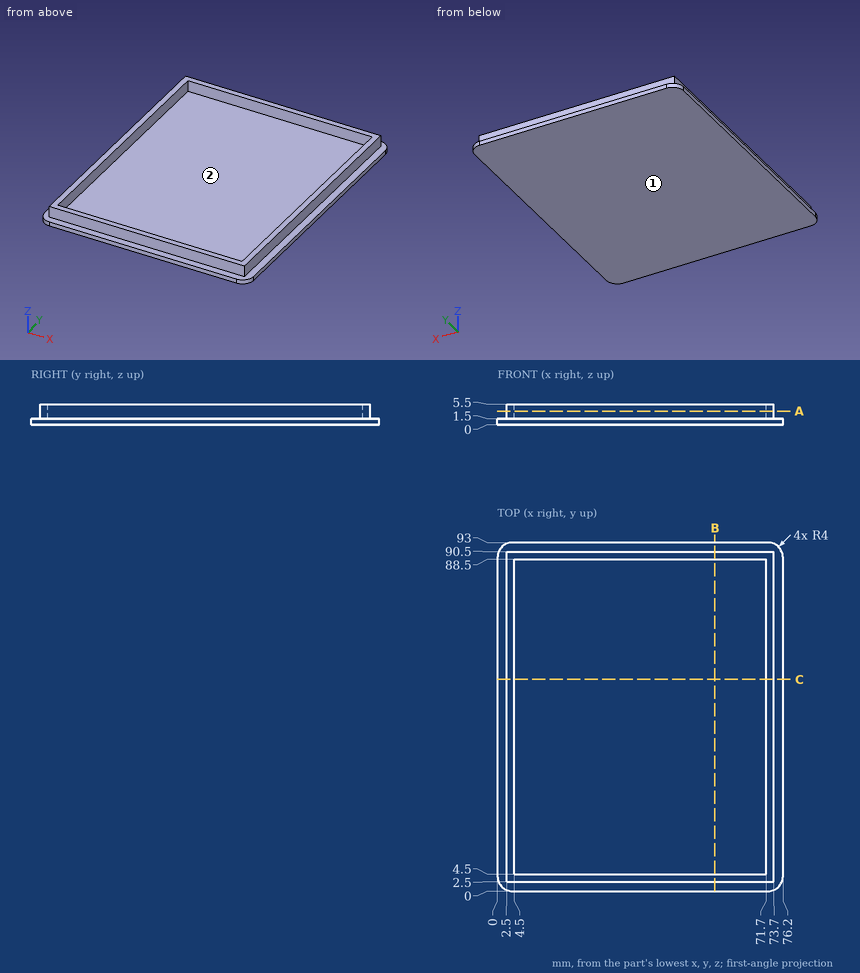
Answer from the drawing. Dimensions are ordinates in mm from the lowest x, y and z of the part. Round coordinates to 2 decimals unless told otherwise and drop trailing zeros. Write each loop counter-clockwise with the first axis right and the second up, starting at its lowest first coordinate (ties: lowest second). Pieces come first, ordered by that corner, then holes. Notation, with made-up numbers: (4.25, 11.5) -> (41.25, 11.5) arc R24 ccw to (41.25, 34.5) -> close; hole circle Ø1 at (-29.5, 4.5). An arc over 180 degrees is marked (long way). Answer in a Markdown table with one row per item. Add a question column.
1) Determine the mould class of the marked faces 1 and 2 for opening direction X: pulls with the +X half, pulls with the -X half, needs draft (parallel to the pull), parting line crosses it, or undercut.
2) Given P1, Ø1.2, axis at y = 49.5, z = 4, coming from the +X side; P2, Ø1.2, axis at x = 43, z = 3.5, coming from the -Y side; P3, Ø2, axis at x = 15.5, y = 82.5, coming from the +Z side, each flat-ended and moving along its own axis, determine where each tip first touches the part or whether it passes through.
3) Find section A-A, the plane z = 3.6. Determine the outline of the cut face in (x, y), and give its area (3 significant figures).
4) Find section B-B, the plane x = 58. Determine the outline of the cut face in (y, z), and give its area (4 significant figures).
5) Find section C-C, the plane y = 56.5. Determine the outline of the cut face in (x, z), and give its area (3 significant figures).
6) Consider line 1 (X direction, y = 13, z = 1.95); line 2 (Y direction, x = 65, z = 4.6); line 3 (Z direction, x = 50, y = 58). Determine where each line is inside the solid, lowest interval first.
Findings below:
| question | item | result |
|---|---|---|
| 1 | face 1 | needs draft |
| 1 | face 2 | undercut |
| 2 | P1 | x = 73.7 |
| 2 | P2 | y = 2.5 |
| 2 | P3 | z = 1.5 |
| 3 | outline | (2.5, 2.5) -> (73.7, 2.5) -> (73.7, 90.5) -> (2.5, 90.5) -> close; hole (4.5, 4.5) -> (71.7, 4.5) -> (71.7, 88.5) -> (4.5, 88.5) -> close |
| 3 | area | 621 mm² |
| 4 | outline | (0, 0) -> (93, 0) -> (93, 1.5) -> (90.5, 1.5) -> (90.5, 5.5) -> (88.5, 5.5) -> (88.5, 1.5) -> (4.5, 1.5) -> (4.5, 5.5) -> (2.5, 5.5) -> (2.5, 1.5) -> (0, 1.5) -> close |
| 4 | area | 155.5 mm² |
| 5 | outline | (0, 0) -> (76.2, 0) -> (76.2, 1.5) -> (73.7, 1.5) -> (73.7, 5.5) -> (71.7, 5.5) -> (71.7, 1.5) -> (4.5, 1.5) -> (4.5, 5.5) -> (2.5, 5.5) -> (2.5, 1.5) -> (0, 1.5) -> close |
| 5 | area | 130 mm² |
| 6 | line 1 | 2.5 to 4.5, 71.7 to 73.7 |
| 6 | line 2 | 2.5 to 4.5, 88.5 to 90.5 |
| 6 | line 3 | 0 to 1.5 |
